Could you check a few things on this model? Use its own coordinates, in mm. A direction names the side the tool comes from. Give positions to 0.01 mm unless a question says otherwise; leave off trailing zeros. Write each loop counter-clockwise with the first axis right and the second up, starting at its lowest first coordinate (ties: lowest second). Pieces come first, ordered by that corner, then holes. Notation, with made-up numbers: (-16, 44) - (17, 44) arc R25 ccw to (17, 69) - close; hole circle Ø1 at (86.5, -20). An arc over 180 degrees is marked (long way). Use one line per item in the form item = value.
```python
from build123d import *

# Parameters (mm, degrees)
SKETCH1_W           = 121
SKETCH1_H           = 80
SKETCH1_W_2         = 20
SKETCH1_H_2         = 5
SKETCH1_W_3         = 12.5
SKETCH1_H_3         = 8.5
BOSS_EXTRUDE1_DEPTH = 4
SKETCH4_R           = 1.185
BOSS_EXTRUDE2_DEPTH = 5


with BuildPart() as part:
    # Sketch1 → Boss-Extrude1 (new body)
    with BuildSketch(Plane(origin=(0, 0, 0), x_dir=(1, 0, 0), z_dir=(0, 1, 0))):
        Rectangle(SKETCH1_W, SKETCH1_H)
        with Locations((39.5, 31.5)):
            Rectangle(SKETCH1_W_2, SKETCH1_H_2, mode=Mode.SUBTRACT)
        Rectangle(SKETCH1_W_3, SKETCH1_H_3, mode=Mode.SUBTRACT)
    extrude(amount=BOSS_EXTRUDE1_DEPTH)

    # Sketch4 → Boss-Extrude2 (add)
    with BuildSketch(Plane.XZ):
        with Locations(Location((-58.5, -38, 0), (0, 0, 270))):
            Circle(SKETCH4_R)
        with Locations(Location((-58.5, 38, 0), (0, 0, 90))):
            Circle(SKETCH4_R)
        with Locations(Location((58.5, -38, 0), (0, 0, 90))):
            Circle(SKETCH4_R)
        with Locations(Location((58.5, 38, 0), (0, 0, 270))):
            Circle(SKETCH4_R)
    extrude(amount=BOSS_EXTRUDE2_DEPTH)


solid = part.part
```
1. Imagine slicing it at D-D, the plane y = -2.75. List the corners of the cut face in (x, z) for me (3 decimals), and give its area (3 significant figures).
Response values:
outline = circle Ø2.37 at (-58.5, -38); circle Ø2.37 at (-58.5, 38); circle Ø2.37 at (58.5, -38); circle Ø2.37 at (58.5, 38)
area = 17.6 mm²
2. If I drill on line 1 (Z direction, x = 40, y = 0.5); line 2 (Y direction, x = 24, z = 3); line 3 (Z direction, x = 0, y = 2.5), over which ranges is the centre line in solid material (lowest first)? Write a range as from..to.
Response values:
line_1 = -40..-34, -29..40
line_2 = 0..4
line_3 = -40..-4.25, 4.25..40
3. Which directions (+Z, -Z, +X, -X, +Y, -Y) give clear straight access to the entire face, cutting with the end or side of a thin tool? Please do faces 5 (the face through (29.5, 2, -31)), 6 (the face through (-1, 2, -40)), 7 (the face through (-59.657, -2.465, -37.743)).
Response values:
face_5 = +Y, -Y
face_6 = -Z, +X, -X, +Y, -Y
face_7 = -Y
4. For pin 1 (6 mm diameter, centred on x = -6.5, z = 30.5, fed in from -Y), with a flat end and sliding along its axis, tell me the tip position at first contact or that it passes through.
Response values:
pin_1 = 0
5. Imagine slicing it at A-A, the plane x = 0. List the corners of the cut face in (y, z) for me.
Response values:
outline = (0, -40) - (4, -40) - (4, -4.25) - (0, -4.25) - close; (0, 4.25) - (4, 4.25) - (4, 40) - (0, 40) - close
6. Imagine slicing it at B-B, the plane z = -38. List the corners of the cut face in (x, y) for me (3 decimals), and give its area (3 significant figures).
Response values:
outline = (-60.5, 0) - (-59.685, 0) - (-59.685, -5) - (-57.315, -5) - (-57.315, 0) - (57.315, 0) - (57.315, -5) - (59.685, -5) - (59.685, 0) - (60.5, 0) - (60.5, 4) - (-60.5, 4) - close
area = 508 mm²
7. If we mould it in two halves opening along X, with no side actions, what happens to faces 1 (the face through (39, 2, -29)), 2 (the face through (-59, -5, 38)), 3 (the face through (60.5, 2, 1)), 4 (the face through (-60.5, 2, 1))? For each: pulls with the +X half, pulls with the -X half, needs draft (parallel to the pull), parting line crosses it, or undercut.
Response values:
face_1 = undercut
face_2 = needs draft
face_3 = pulls with the +X half
face_4 = pulls with the -X half
8. Imagine slicing it at C-C, the plane x = 58.5. List the corners of the cut face in (y, z) for me (3 decimals), and give its area (3 significant figures).
Response values:
outline = (-5, -39.185) - (0, -39.185) - (0, -40) - (4, -40) - (4, 40) - (0, 40) - (0, 39.185) - (-5, 39.185) - (-5, 36.815) - (0, 36.815) - (0, -36.815) - (-5, -36.815) - close
area = 344 mm²
